Geometry check sheet. Reference: the model listing, model coordinates, mm. A direction names the side the tool comes from. Round coordinates to 2 decimals unless told otherwise and drop trailing zeros. Write each loop counter-clockwise with the first axis right and the second up, starting at its lowest first coordinate (ties: lowest second). Pieces come first, ordered by that corner, then holes. Notation, with made-up numbers: (-29.5, 34.25) -> (-2.5, 34.25) arc R31 ccw to (-2.5, 60.25) -> close; hole circle Ø9 at (-6, 65.25). An arc over 180 degrees is marked (long way). Put each result on its own line as item: value. Start each with the question number.
from build123d import *

# Parameters (mm, degrees)
BOSS_EXTRUDE1_DEPTH = 26
BOSS_EXTRUDE2_DEPTH = 4


with BuildPart() as part:
    # Sketch1 → Boss-Extrude1 (new, symmetric)
    with BuildSketch(Plane.XY):
        with BuildLine():
            Line((0, 35.584487251), (0, 0))
            Line((0, 0), (37.5, 0))
            Line((37.5, 0), (37.5, 9))
            Line((37.5, 9), (4.5, 9))
            Line((4.5, 9), (4.5, 26.444512863))
            ThreePointArc((4.5, 26.444512863), (17.783419244, 34.414047854), (23, 49))
            Line((23, 49), (13.415512749, 49))
            ThreePointArc((13.415512749, 49), (9.486200038, 39.513799962), (0, 35.584487251))
        make_face()
        with BuildLine():
            Line((-37.5, 9), (-37.5, 0))
            Line((-37.5, 0), (0, 0))
            Line((0, 0), (0, 35.584487251))
            ThreePointArc((0, 35.584487251), (-9.486200038, 39.513799962), (-13.415512749, 49))
            Line((-13.415512749, 49), (-23, 49))
            ThreePointArc((-23, 49), (-17.783419244, 34.414047854), (-4.5, 26.444512863))
            Line((-4.5, 26.444512863), (-4.5, 9))
            Line((-4.5, 9), (-37.5, 9))
        make_face()
    extrude(amount=BOSS_EXTRUDE1_DEPTH, both=True)

    # Sketch1_3 → Boss-Extrude2 (add, symmetric)
    with BuildSketch(Plane.XY):
        with BuildLine():
            ThreePointArc((4.5, 26.444512863), (17.783419244, 34.414047854), (23, 49))
            Line((23, 49), (37.5, 9))
            Line((37.5, 9), (4.5, 9))
            Line((4.5, 9), (4.5, 26.444512863))
        make_face()
        with BuildLine():
            Line((-4.5, 9), (-4.5, 26.444512863))
            ThreePointArc((-4.5, 26.444512863), (-17.783419244, 34.414047854), (-23, 49))
            Line((-23, 49), (-37.5, 9))
            Line((-37.5, 9), (-4.5, 9))
        make_face()
    extrude(amount=BOSS_EXTRUDE2_DEPTH, both=True)


solid = part.part
(1) Material ranges on L1, parallel to X at y = 16, z = 15.5; L2, parallel to Z at x = 18, y = 11.5; L3, parallel to Y at x = 25, z = -16, recorded low to high. Write a range as from..to.
(2) Sectioned sample at B-B (z = -19). Record the cut outline in (x, y).
(3) Sectioned sample at C-C (y = 45.5). Record the cut outline in (x, z).
(4) Sectioned sample at D-D (x = 0). Record the cut outline in (y, z).
(5) Go/stop test with flat-tipped pins: pin 1 Ø5 at (y, z) = (13.5, 16) entering from -X; pin 2 Ø1 at (x, z) = (7.5, 19) entering from +Y; pin 3 Ø5 at (y, z) = (41.5, -2.5) entering from -X (3 decimals). Record where each tip stops, or that it passes through.
(6) Set-up check for faces 4 (the flat face through (-18, 49, 0)), 5 (the flat face through (4.5, 18, 15)), 6 (the flat face through (4.5, 18, -15)), 7 (the cylindrical face through (-17.923, 34.586, 15.154)), 8 (the cylindrical face through (-17.923, 34.586, -14.846)): record each of +Z, -Z, +X, -X, +Y, -Y from which the full face is reachable in a straight line by a thin tool's end or side.
(7) Sectioned sample at A-A (y = 21). Record the cut outline in (x, z).
(8) Mould release check, pull along X, two halves, no side actions. Record for faces 1 (the flat face through (-30.15, 29.28, 0.06)), 2 (the flat face through (21, 20, -4)), 3 (the cylindrical face through (0.295, 35.588, 0.364)): +X half, -X half, draft (parallel to the pull), parting line (faces both ways), or undercut.
Found:
1. L1: -4.5..4.5
1. L2: -4..4
1. L3: 0..9
2. outline: (-37.5, 0) -> (37.5, 0) -> (37.5, 9) -> (4.5, 9) -> (4.5, 26.44) arc R23 ccw to (23, 49) -> (13.42, 49) arc R13.42 cw to (-13.42, 49) -> (-23, 49) arc R23 ccw to (-4.5, 26.44) -> (-4.5, 9) -> (-37.5, 9) -> close
3. outline: (-24.27, -4) -> (-22.73, -4) -> (-22.73, -26) -> (-12.95, -26) -> (-12.95, 26) -> (-22.73, 26) -> (-22.73, 4) -> (-24.27, 4) -> close; (12.95, -26) -> (22.73, -26) -> (22.73, -4) -> (24.27, -4) -> (24.27, 4) -> (22.73, 4) -> (22.73, 26) -> (12.95, 26) -> close
4. outline: (0, -26) -> (35.58, -26) -> (35.58, 26) -> (0, 26) -> close
5. pin 1: x = -4.5
5. pin 2: y = 38.23
5. pin 3: x = -26.625
6. face 4: +Z, -Z, +X, -X, +Y
6. face 5: +Z, +X
6. face 6: -Z, +X
6. face 7: +Z, -X
6. face 8: -Z, -X
7. outline: (-33.15, -4) -> (-4.5, -4) -> (-4.5, -26) -> (4.5, -26) -> (4.5, -4) -> (33.15, -4) -> (33.15, 4) -> (4.5, 4) -> (4.5, 26) -> (-4.5, 26) -> (-4.5, 4) -> (-33.15, 4) -> close
8. face 1: -X half
8. face 2: draft
8. face 3: undercut
